```python
from build123d import *

# Parameters (mm, degrees)
SKETCH2_W           = 50
SKETCH2_H           = 30
BOSS_EXTRUDE1_DEPTH = 4
SKETCH3_R           = 10.75
BOSS_EXTRUDE2_DEPTH = 4
SKETCH4_R           = 10.75
SKETCH4_R_2         = 6.25
BOSS_EXTRUDE3_DEPTH = 1
SKETCH5_R           = 6.25
SKETCH5_R_2         = 5.01
BOSS_EXTRUDE4_DEPTH = 1
BOSS_EXTRUDE5_START = -1
SKETCH6_R           = 6.25
SKETCH6_R_2         = 4.875
BOSS_EXTRUDE5_DEPTH = 1
SKETCH8_R           = 0.875
CUT_EXTRUDE1_DEPTH  = 10


with BuildPart() as part:
    # Sketch2 → Boss-Extrude1 (new body)
    with BuildSketch(Plane(origin=(0, 0, 0), x_dir=(1, 0, 0), z_dir=(0, 1, 0))):
        Rectangle(SKETCH2_W, SKETCH2_H)
    extrude(amount=BOSS_EXTRUDE1_DEPTH)

    # Sketch3 → Boss-Extrude2 (add)
    with BuildSketch(Plane.ZY.offset(25)):
        with BuildLine():
            Line((-15, 0), (-15, 35))
            ThreePointArc((-15, 35), (0, 50), (15, 35))
            Line((15, 35), (15, 0))
            Line((15, 0), (-15, 0))
        make_face()
        with Locations((0, 35)):
            Circle(SKETCH3_R, mode=Mode.SUBTRACT)
    boss_extrude2 = extrude(amount=BOSS_EXTRUDE2_DEPTH)

    # Mirror1: Boss-Extrude2 across plane
    add(boss_extrude2.mirror(Plane(origin=(0, 0, 0), x_dir=(0, 0, 1), z_dir=(1, 0, 0))))

    # Sketch4 → Boss-Extrude3 (add)
    with BuildSketch(Plane(origin=(-25, 0, 0), x_dir=(0, 0, -1), z_dir=(1, 0, 0))):
        with Locations((0, 35)):
            Circle(SKETCH4_R)
        with Locations((0, 35)):
            Circle(SKETCH4_R_2, mode=Mode.SUBTRACT)
    boss_extrude3 = extrude(amount=-BOSS_EXTRUDE3_DEPTH)

    # Mirror2: Boss-Extrude3 across plane
    add(boss_extrude3.mirror(Plane(origin=(0, 0, 0), x_dir=(0, 0, 1), z_dir=(1, 0, 0))))

    # Sketch5 → Boss-Extrude4 (add)
    with BuildSketch(Plane(origin=(26, 0, 0), x_dir=(0, 0, -1), z_dir=(1, 0, 0))):
        with Locations((0, 35)):
            Circle(SKETCH5_R)
        with Locations((0, 35)):
            Circle(SKETCH5_R_2, mode=Mode.SUBTRACT)
    extrude(amount=-BOSS_EXTRUDE4_DEPTH)

    # Sketch6 → Boss-Extrude5 (add)
    with BuildSketch(Plane.ZY.offset(26).offset(BOSS_EXTRUDE5_START)):
        with Locations((0, 35)):
            Circle(SKETCH6_R)
        with Locations((0, 35)):
            Circle(SKETCH6_R_2, mode=Mode.SUBTRACT)
    extrude(amount=BOSS_EXTRUDE5_DEPTH)

    # Sketch8 → Cut-Extrude1 (cut)
    with BuildSketch(Plane.XZ):
        with Locations(Location((-6.75, 6.75, 0), (0, 0, 270))):
            Circle(SKETCH8_R)
        with Locations(Location((6.75, 6.75, 0), (0, 0, 270))):
            Circle(SKETCH8_R)
        with Locations(Location((6.75, -6.75, 0), (0, 0, 270))):
            Circle(SKETCH8_R)
        with Locations(Location((-6.75, -6.75, 0), (0, 0, 270))):
            Circle(SKETCH8_R)
    extrude(amount=-CUT_EXTRUDE1_DEPTH, mode=Mode.SUBTRACT)


solid = part.part
```
Input: part model. Units: mm. Frame: model coordinates. A direction names the side the tool comes from. Give positions to 0.01 mm unless a question says otherwise; leave off trailing zeros. Write each loop counter-clockwise with the first axis right and the second up, starting at its lowest first coordinate (ties: lowest second). Pieces come first, ordered by that corner, then holes. Notation, with made-up numbers: (43, 53) - (97, 53) arc R23 ccw to (97, 89) - close; hole circle Ø7 at (11.25, 4.25). An arc over 180 degrees is marked (long way). Write item = value, one per line. Start each with the question number.
1. Section query D-D, the plane y = 36. Output: boundary loops of the cut face in (x, z).
2. Section query A-A, the plane y = 9. Output: boundary loops of the cut face in (x, z).
3. Section query C-C, the plane z = 0. Output: boundary loops of the cut face in (x, y) (3 decimals).
4. Ray query, L1, parallel to X at y = 2.2, z = 6.75 (3 decimals); L2, parallel to Y at x = -28, z = 0; L3, parallel to Z at x = 27.7, y = 35. Return the intervals inside material, ascending.
5. First-contact query: pin 1 Ø10 at (x, z) = (16.5, -8.5) entering from +Y; pin 2 Ø13 at (y, z) = (35, 0) entering from -X; pin 3 Ø6 at (y, z) = (34.5, 3.5) entering from +X. Flat tips, straight axial feed; report the tip coordinate or a pass-through.
6. Access query for faces 1 (the flat face through (0, 4, 0)), 2 (the cylindrical face through (7.5, 2, 6.3)), 3 (the flat face through (-26, 30, 2)). Directions: +Z, -Z, +X, -X, +Y, -Y. A direction counts if a zero-diameter tool reaches every point of the face in a straight line with its end or side. Return the directions, or none.
7. Mould query, pull axis Y, two halves, no side actions, for faces 4 (the cylindrical face through (25.51, 30.11, 1.09)), 5 (the flat face through (0, 0, 0)), 6 (the cylindrical face through (-27, 50, 0)), 7 (the cylindrical face through (7.5, 2, -7.2)). Classes: released by +Y, released by -Y, zero draft, split by the parting line, or undercut.
8. Section query B-B, the plane x = 6.75. Output: boundary loops of the cut face in (y, z) (3 decimals).
Check sheet entries:
q1.outline = (-29, -14.97) - (-25, -14.97) - (-25, -4.77) - (-26, -4.77) - (-26, -10.7) - (-29, -10.7) - close; (-29, 10.7) - (-26, 10.7) - (-26, 4.77) - (-25, 4.77) - (-25, 14.97) - (-29, 14.97) - close; (25, -14.97) - (29, -14.97) - (29, -10.7) - (26, -10.7) - (26, -4.91) - (25, -4.91) - close; (25, 4.91) - (26, 4.91) - (26, 10.7) - (29, 10.7) - (29, 14.97) - (25, 14.97) - close
q2.outline = (-29, -15) - (-25, -15) - (-25, 15) - (-29, 15) - close; (25, -15) - (29, -15) - (29, 15) - (25, 15) - close
q3.outline = (-29, 0) - (29, 0) - (29, 24.25) - (26, 24.25) - (26, 29.99) - (25, 29.99) - (25, 4) - (-25, 4) - (-25, 30.125) - (-26, 30.125) - (-26, 24.25) - (-29, 24.25) - close; (-29, 45.75) - (-26, 45.75) - (-26, 39.875) - (-25, 39.875) - (-25, 50) - (-29, 50) - close; (25, 40.01) - (26, 40.01) - (26, 45.75) - (29, 45.75) - (29, 50) - (25, 50) - close
q4.L1 = -29 to -7.625, -5.875 to 5.875, 7.625 to 29
q4.L2 = 0 to 24.25, 45.75 to 50
q4.L3 = -15 to -10.75, 10.75 to 15
q5.pin_1 = 4
q5.pin_2 = -26
q5.pin_3 = 26
q6.face_1 = +Z, -Z, +Y
q6.face_2 = +Y, -Y
q6.face_3 = -X
q7.face_4 = undercut
q7.face_5 = released by -Y
q7.face_6 = released by +Y
q7.face_7 = zero draft
q8.outline = (0, -15) - (4, -15) - (4, -7.625) - (0, -7.625) - close; (0, -5.875) - (4, -5.875) - (4, 5.875) - (0, 5.875) - close; (0, 7.625) - (4, 7.625) - (4, 15) - (0, 15) - close
